```python
from build123d import *

# Parameters (mm, degrees)
F0_R          = 20
F0_R_2        = 12.7
F0_R_3        = 9
F1_DEPTH      = 47
F2_DEPTH      = 77
F3_DEPTH      = 40
F5_DEPTH      = 15.5956
F7_START      = 5.8
F7_DEPTH      = 3.2
F9_DEPTH      = 0.8
F9_DEPTH_BACK = 25


with BuildPart() as f1:
    # F0 (on Top) → F1 (new body)
    with BuildSketch(Plane.XY):
        Circle(F0_R)
        Circle(F0_R_2, mode=Mode.SUBTRACT)
        Circle(F0_R_2)
        Circle(F0_R_3, mode=Mode.SUBTRACT)
    extrude(amount=F1_DEPTH)

    # F0 (on Top) → F2 (join)
    with BuildSketch(Plane.XY):
        Circle(F0_R_3)
    extrude(amount=F2_DEPTH)

    # F0 (on Top) → F3 (cut)
    with BuildSketch(Plane.XY):
        Circle(F0_R_2)
        Circle(F0_R_3, mode=Mode.SUBTRACT)
        Circle(F0_R_3)
    extrude(amount=F3_DEPTH, mode=Mode.SUBTRACT)

    # F4 (on Front) → F5 (cut)
    with BuildSketch(Plane.XZ):
        Polygon((-3.175, 0), (0, 0), (3.175, 0), (3.175, 40), (-3.175, 40), align=None)
    extrude(amount=F5_DEPTH, mode=Mode.SUBTRACT)

    # F6 (on Front) → F7 (cut)
    with BuildSketch(Plane.XZ.offset(F7_START)):
        with BuildLine():
            Line((3, 53.5), (3, 70.5))
            ThreePointArc((3, 70.5), (0, 67.5), (-3, 70.5))
            Line((-3, 70.5), (-3, 53.5))
            ThreePointArc((-3, 53.5), (0, 56.5), (3, 53.5))
        make_face()
        with BuildLine():
            ThreePointArc((0, 50.5), (2.1213203436, 51.3786796564), (3, 53.5))
            ThreePointArc((3, 53.5), (0, 56.5), (-3, 53.5))
            ThreePointArc((-3, 53.5), (-2.1213203436, 51.3786796564), (0, 50.5))
        make_face()
        with BuildLine():
            ThreePointArc((3, 70.5), (2.1213203436, 72.6213203436), (0, 73.5))
            ThreePointArc((0, 73.5), (-2.1213203436, 72.6213203436), (-3, 70.5))
            ThreePointArc((-3, 70.5), (0, 67.5), (3, 70.5))
        make_face()
    extrude(amount=F7_DEPTH, mode=Mode.SUBTRACT)

    # F8 (on Front) → F9 (cut, two sides)
    with BuildSketch(Plane.XZ) as f9_sk:
        with BuildLine():
            ThreePointArc((0, 5.5), (1.767766953, 6.232233047), (2.5, 8))
            ThreePointArc((2.5, 8), (1.767766953, 9.767766953), (0, 10.5))
            Line((0, 10.5), (0, 8))
            Line((0, 8), (0, 5.5))
        make_face()
        with BuildLine():
            ThreePointArc((2.5, 32), (-1.767766953, 33.767766953), (0, 29.5))
            ThreePointArc((0, 29.5), (1.767766953, 30.232233047), (2.5, 32))
        make_face()
        with BuildLine():
            Line((0, 8), (0, 10.5))
            ThreePointArc((0, 10.5), (-2.5, 8), (0, 5.5))
            Line((0, 5.5), (0, 8))
        make_face()
    extrude(amount=-F9_DEPTH, mode=Mode.SUBTRACT)
    extrude(f9_sk.sketch, amount=F9_DEPTH_BACK, mode=Mode.SUBTRACT)


solid = f1.part
```
Work out the finished part from the listing and answer in its coordinate system (mm). A direction names the side the tool comes from. Round coordinates to 2 decimals unless told otherwise and drop trailing zeros. Loops run counter-clockwise (first coordinate to the right, second up) from the corner with the lowest first, then second, coordinate; pieces in that order, holes last. Notation, with made-up numbers: (-9, 17) -> (42, 17) arc R12 cw to (42, 30) -> close; hole circle Ø5 at (52, 80.5). An arc over 180 degrees is marked (long way). Write each question's results on one line, items separated by ' | '. Start each with the question number.
1. Section B-B (y = 0) is taken. Determine the outline of the cut face in (x, z), plus the area to 3 significant figures.
2. A tool of negligible diameter and unlimited length cuts with its end or side. For faces 1 (the face through (0, -15.596, 20)), 2 (the face through (9, -4, 47)), 3 (the face through (3, -7, 62)), 4 (the face through (0, 0, 77)), from which of +Z, -Z, +X, -X, +Y, -Y can it reach the whole face along a straight path? Write none if from no direction.
3. Section D-D (z = 69.5) is taken. Determine the outline of the cut face in (x, y), plus the area to 3 significant figures.
4. Find the intervals of material crossed by probe 1 along Z at (x, y) = (-2, 15.5); probe 2 along Y at (x, z) = (6.5, 17); probe 3 along Z at (x, y) = (-9.5, 6), in increasing order. Write a range as from..to.
5. For a pull along X with two mould halves and no side action, classify faces 5 (the face through (0, -1, 40)), 6 (the face through (-4.336, -19.524, 23.171)), 7 (the face through (13, 0, 0)) as +X half, -X half, draft (parallel to the pull), parting line (faces both ways), or undercut.
6. Section A-A (z = 38) is taken. Determine the outline of the cut face in (x, y) (3 decimals).
7. Section C-C (y = -17) is taken. Determine the outline of the cut face in (x, z), plus the area to 3 significant figures.
8. Given pin 1 Ø3 at (x, z) = (-1.5, 15.5) entering from +Y; pin 2 Ø1 at (y, z) = (-4, 11) entering from -X; pin 3 Ø0.8 at (y, z) = (-6.5, 64.5) entering from +X, each flat-ended and moving along its own axis, determine where each tip first touches the part or whether it passes through.
Evaluation:
1) outline: (-20, 0) -> (-12.7, 0) -> (-12.7, 40) -> (12.7, 40) -> (12.7, 0) -> (20, 0) -> (20, 47) -> (9, 47) -> (9, 77) -> (-9, 77) -> (-9, 47) -> (-20, 47) -> close | area: 1,400 mm2
2) face 1: -Z | face 2: +Z | face 3: -Y | face 4: +Z, +X, -X, +Y, -Y
3) outline: (-3, -8.49) -> (-3, -5.8) -> (3, -5.8) -> (3, -8.49) arc R9 ccw (long way) to start | area: 236 mm2
4) probe 1: z = 0..47 | probe 2: y = -18.91..-10.91, 10.91..18.91 | probe 3: z = 40..47
5) face 5: undercut | face 6: parting line | face 7: draft
6) outline: circle Ø40 at (0, 0); hole (-3.175, -15.596) -> (3.175, -15.596) -> (3.175, -12.297) arc R12.7 ccw (long way) to (-3.175, -12.297) -> close
7) outline: (-10.54, 0) -> (10.54, 0) -> (10.54, 47) -> (-10.54, 47) -> close; hole circle Ø5 at (0, 8); hole circle Ø5 at (0, 32) | area: 951 mm2
8) pin 1: stops at y = 20 | pin 2: stops at x = -19.69 | pin 3: stops at x = 6.62
